The model under review builds one solid part; all positions refer to its coordinate system, in mm. Give positions to 0.01 mm unless a question says otherwise; leave off trailing zeros. Return JSON: item names as keys, results as strings. Group by question number.
from build123d import *

# Parameters (mm, degrees)
SKETCH1_W           = 131.318
SKETCH1_H           = 148.082
BOSS_EXTRUDE1_DEPTH = 3
SKETCH2_R           = 2.25
CUT_EXTRUDE1_DEPTH  = 4
FILLET1_R           = 5


with BuildPart() as part:
    # Sketch1 → Boss-Extrude1 (new body)
    with BuildSketch(Plane(origin=(0, 0, 0), x_dir=(1, 0, 0), z_dir=(0, 1, 0))):
        with Locations((0.406931424, 0.203465712)):
            Rectangle(SKETCH1_W, SKETCH1_H)
    extrude(amount=BOSS_EXTRUDE1_DEPTH)

    # Sketch2 → Cut-Extrude1 (cut, through all)
    with BuildSketch(Plane(origin=(0, 3, 0), x_dir=(1, 0, 0), z_dir=(0, 1, 0))):
        with Locations((-56.934068576, -65.755534288)):
            Circle(SKETCH2_R)
        with Locations((-56.934068576, 66.244465712)):
            Circle(SKETCH2_R)
        with Locations((58.065931424, 66.244465712)):
            Circle(SKETCH2_R)
        with Locations((58.065931424, -65.755534288)):
            Circle(SKETCH2_R)
    extrude(amount=-CUT_EXTRUDE1_DEPTH, mode=Mode.SUBTRACT)

    # Fillet1
    fillet1_edges = [part.edges().sort_by_distance(p)[0] for p in [
        (-65.252068576, 1.5, 73.837534288),
        (-65.252068576, 1.5, -74.244465712),
        (66.065931424, 1.5, -74.244465712),
        (66.065931424, 1.5, 73.837534288),
    ]]
    fillet(fillet1_edges, radius=FILLET1_R)


solid = part.part
Item 1: For L1, parallel to Z at x = -55, y = 2.5; L2, parallel to X at y = 2.15, z = -67.5, list the stretches that pass through material, from the lowest coordinate up. Write a range as from..to.
Item 2: For P1, Ø4, axis at x = -56.93, z = 65.76, coming from the -Y side, flat-tipped, find the tip position at first contact; note if it passes through.
Item 3: Mouldability with a two-part tool opening along Z and no side actions: class faces 1 (the face through (60.212, 1.521, 65.08)), 2 (the face through (-63.826, 1.521, -72.741)), 3 (the face through (66.066, 1, 1)) as +Z half, -Z half, draft (parallel to the pull), parting line (faces both ways), or undercut.
Check sheet entries:
{
 "1": {"L1": "z = -74.24..-67.39, -65.09..64.61, 66.91..73.84", "L2": "x = -65.25..-58.8, -55.07..56.2, 59.93..66.07"},
 "2": {"P1": "passes through"},
 "3": {"face 1": "undercut", "face 2": "-Z half", "face 3": "draft"}
}
